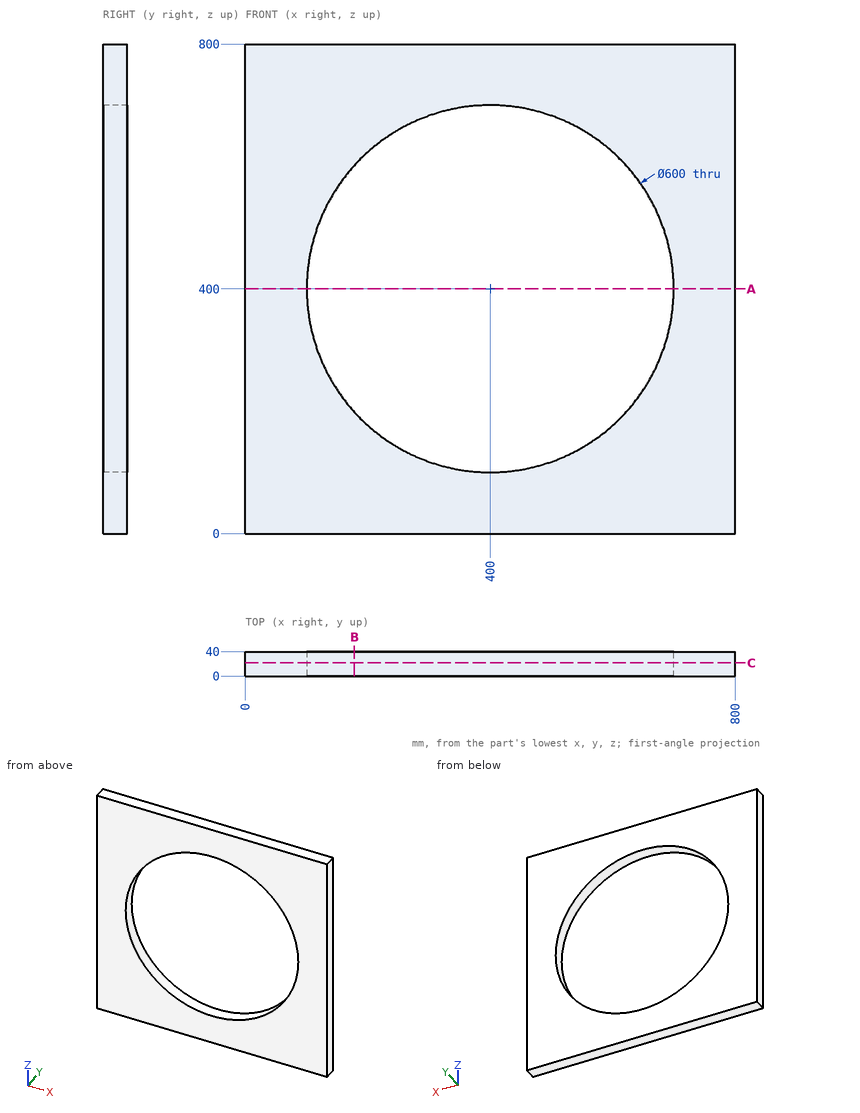
Drawing for the job (mm, zero at the part's lowest x, y, z). Give positions to 0.01 mm unless a question says otherwise; leave off trailing zeros. Loops run counter-clockwise (first coordinate to the right, second up) from the corner with the lowest first, then second, coordinate; pieces in that order, holes last.
Item 1: Slice it at C-C (y = 21.5). Write the cut outline in (x, z).
Check values:
outline: (0, 0) - (800, 0) - (800, 800) - (0, 800) - close; hole circle Ø600 at (400, 400)
Item 2: Drill centre lines: line 1 along Z through (x, y) = (400, 24); line 2 along X through (y, z) = (34, 554); line 3 along X through (y, z) = (36, 382). Where is each one in solid material? Low to high.
Check values:
line 1: z = 0 to 100, 700 to 800
line 2: x = 0 to 142.54, 657.46 to 800
line 3: x = 0 to 100.54, 699.46 to 800
Item 3: Slice it at A-A (z = 400). Write the cut outline in (x, y), plus the area to 3 significant figures.
Check values:
outline: (0, 0) - (100, 0) - (100, 40) - (0, 40) - close; (700, 0) - (800, 0) - (800, 40) - (700, 40) - close
area: 8,000 mm2
Item 4: Slice it at B-B (x = 178). Write the cut outline in (y, z).
Check values:
outline: (0, 0) - (40, 0) - (40, 198.22) - (0, 198.22) - close; (0, 601.78) - (40, 601.78) - (40, 800) - (0, 800) - close
